The model under review builds one solid part; all positions refer to its coordinate system, in mm. Face numbers are marked on the shaded views. Round coordinates to 2 decimals unless told otherwise and drop trailing zeros. Write each loop counter-clockwise with the first axis right and the second up, starting at its lowest first coordinate (ties: lowest second). Pieces come first, ordered by that corner, then holes. Notation, with made-up numbers: (17, 54) - (65, 54) arc R17 ccw to (65, 66) - close; hole circle Ø5 at (14.25, 66.25). An arc over 180 degrees is marked (long way). Write each question's results on one line, items separated by ' | '.
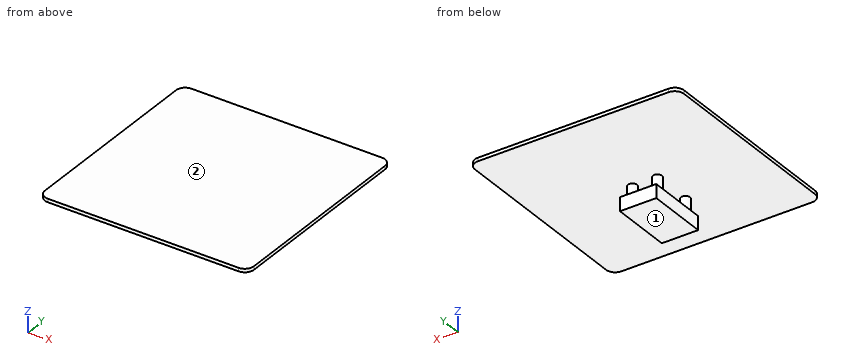
```python
from build123d import *

# Parameters (mm, degrees)
F1_DEPTH = 4.826
F2_R     = 6.35
F3_DEPTH = 19.05
F5_W     = 50.8
F5_H     = 85.09
F6_DEPTH = 19.05


with BuildPart() as f1:
    # F0 (on Top) → F1 (new body)
    with BuildSketch(Plane.XY):
        with BuildLine():
            ThreePointArc((146.05, 133.35), (142.330256, 142.330256), (133.35, 146.05))
            Line((133.35, 146.05), (-133.35, 146.05))
            ThreePointArc((-133.35, 146.05), (-142.330256, 142.330256), (-146.05, 133.35))
            Line((-146.05, 133.35), (-146.05, -133.35))
            ThreePointArc((-146.05, -133.35), (-142.330256, -142.330256), (-133.35, -146.05))
            Line((-133.35, -146.05), (133.35, -146.05))
            ThreePointArc((133.35, -146.05), (142.330256, -142.330256), (146.05, -133.35))
            Line((146.05, -133.35), (146.05, 133.35))
        make_face()
    extrude(amount=F1_DEPTH)

    # F2 (on Top) → F3 (join)
    with BuildSketch(Plane.XY):
        with Locations((-17.399, -57.15)):
            Circle(F2_R)
        with Locations((17.399, -57.15)):
            Circle(F2_R)
        with Locations((17.399, 0)):
            Circle(F2_R)
        with Locations((-17.399, 0)):
            Circle(F2_R)
    extrude(amount=-F3_DEPTH)

    # F5 (on offset) → F6 (join)
    with BuildSketch(Plane.XY.offset(-19.05)):
        with Locations((0, -28.575)):
            Rectangle(F5_W, F5_H)
    extrude(amount=-F6_DEPTH)


solid = f1.part
```
Q1. For probe 1 along Z at (x, y) = (-113, -78.5); probe 2 along X at (y, z) = (-56, -5); probe 3 along X at (y, z) = (-40.5, -28.5), list the stretches that pass through material, from the lowest coordinate up.
Evaluation:
probe 1: z = 0 to 4.83 | probe 2: x = -23.64 to -11.15, 11.15 to 23.64 | probe 3: x = -25.4 to 25.4
Q2. We need section C-C (x = -90). State the section outline as (y, z) points, plus the area to 3 significant figures.
Evaluation:
outline: (-146.05, 0) - (146.05, 0) - (146.05, 4.83) - (-146.05, 4.83) - close | area: 1,410 mm^2
Q3. The part is to be moulded in two halves that separate along Z. For the marked faces 1 and 2, say which applies: released by +Z, released by -Z, zero draft, split by the parting line, or undercut.
Evaluation:
face 1: released by -Z | face 2: released by +Z
Q4. We need section B-B (z = -15). State the section outline as (x, y) points, plus the area to 3 significant figures.
Evaluation:
outline: circle Ø12.7 at (-17.4, -57.15); circle Ø12.7 at (-17.4, 0); circle Ø12.7 at (17.4, -57.15); circle Ø12.7 at (17.4, 0) | area: 507 mm^2
Q5. Insertion check: P1, Ø5.5, axis at x = -1.5, z = -30, coming from the -Y side; P2, Ø9.5, axis at y = -35.5, z = -27, coming from the +X side; P3, Ø15, axis at y = -21, z = -26, coming from the -X side. Each pin has a flat end and moves straight along its axis. Give the tip position at first contact, or say it passes through.
Evaluation:
P1: stops at y = -71.12 | P2: stops at x = 25.4 | P3: stops at x = -25.4
Q6. We need section D-D (z = -32). State the section outline as (x, y) points.
Evaluation:
outline: (-25.4, -71.12) - (25.4, -71.12) - (25.4, 13.97) - (-25.4, 13.97) - close
Q7. We need section A-A (y = 0). State the section outline as (x, z) points.
Evaluation:
outline: (-146.05, 0) - (-23.75, 0) - (-23.75, -19.05) - (-25.4, -19.05) - (-25.4, -38.1) - (25.4, -38.1) - (25.4, -19.05) - (23.75, -19.05) - (23.75, 0) - (146.05, 0) - (146.05, 4.83) - (-146.05, 4.83) - close; hole (-11.05, -19.05) - (11.05, -19.05) - (11.05, 0) - (-11.05, 0) - close
